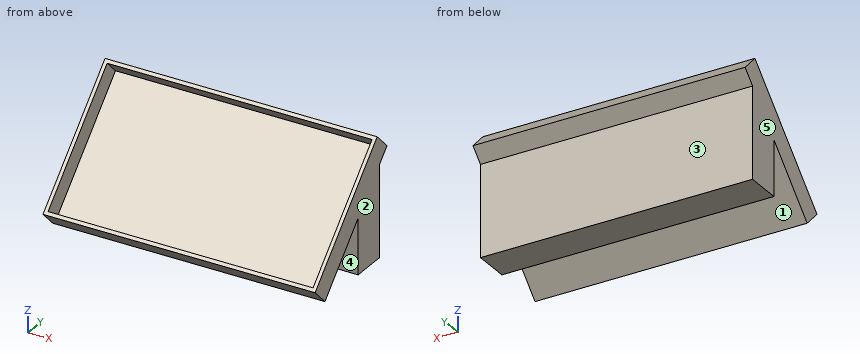
from build123d import *

# Parameters (mm, degrees)
F1_DEPTH = 152
F2_T     = -2
F4_DEPTH = 152


with BuildPart() as f1:
    # F0 (on Right) → F1 (new body)
    with BuildSketch(Plane.YZ):
        Polygon((24.395184, 33.587572), (-33.587572, -24.395184), (-24.395184, -33.587572), (33.587572, 24.395184), align=None)
    extrude(amount=F1_DEPTH)

    # F2
    f2_openings = [f1.faces().sort_by_distance(p)[0] for p in [
        (76, -4.596194, 4.596194),
    ]]
    offset(amount=F2_T, openings=f2_openings)

    # F3 (on Right) → F4 (join)
    with BuildSketch(Plane.YZ):
        Polygon((7.990418, 0), (6.604816, 0), (6.604816, -33.587572), (26.604816, -33.587572), (26.604816, 0), align=None)
        Polygon((26.604816, 18.73309), (7.990418, 0), (26.604816, 0), align=None)
    extrude(amount=F4_DEPTH)


solid = f1.part
Could you check a few things on this model? Use its own coordinates, in mm. Face numbers are marked on the shaded views. A direction names the side the tool comes from. Give positions to 0.01 mm unless a question says otherwise; leave off trailing zeros. Order: outer loops, then holes, each group sorted by start corner. A loop starts at its lowest first (then second) coordinate and runs counter-clockwise, first axis right, second up. Notation, with made-up numbers: (-21, 78.5) - (-4, 78.5) arc R23 cw to (-4, 90.5) - close; hole circle Ø5 at (14, 27.25). An arc over 180 degrees is marked (long way). One line per item, written item: value. Start each with the question number.
1. Thinking about a two-plate mould opening in Y: for the marked faces 1, 2 and 3, which applies, +Y half, -Y half, draft (parallel to the pull), parting line (faces both ways), or undercut?
2. For P1, Ø1.5, axis at x = 133, y = -18.5, coming from the +Z side; P2, Ø10, axis at x = 72.5, y = 6.5, coming from the +Z side; P3, Ø4, axis at x = 37.5, z = -9, coming from the +Y side, each with a flat end and sliding along its axis, tell me the tip position at first contact or that it passes through.
3. Imagine slicing it at B-B on x = 112.5. List the corners of the cut face in (y, z) for me, plus the area to 3 significant figures.
4. If I drill on probe 1 along X at (y, z) = (12.5, 19); probe 2 along Y at (x, z) = (99, -26); probe 3 along Z at (x, y) = (127.5, 27), over which ranges is the centre line in solid material (lowest first)?
5. Imagine slicing it at D-D on y = 16.5. List the corners of the cut face in (x, z) for me.
6. Imagine slicing it at C-C on z = 21. List the corners of the cut face in (x, y) for me, plus the area to 3 significant figures.
7. For the marked faces 4 and 5, which set-ups out of +Z, -Z, +X, -X, +Y, -Y let a thin tool reach every point of the face, with its end or its side?
8. Imagine slicing it at A-A on z = -11.5. List the corners of the cut face in (x, y) for me, plus the area to 3 significant figures.
Values:
1. face 1: undercut
1. face 2: draft
1. face 3: +Y half
2. P1: z = -24.11
2. P2: z = 5.14
2. P3: y = 26.6
3. outline: (-33.59, -24.4) - (-24.4, -33.59) - (6.6, -2.59) - (6.6, -33.59) - (26.6, -33.59) - (26.6, 17.41) - (33.59, 24.4) - (24.4, 33.59) - (22.98, 32.17) - (30.76, 24.4) - (-24.4, -30.76) - (-32.17, -22.98) - close
3. area: 1,030 mm²
4. probe 1: 0 to 2, 150 to 152
4. probe 2: -31.98 to -29.15, -19.64 to -16.81, 6.6 to 26.6
4. probe 3: 17.81 to 20.64, 28.15 to 30.98
5. outline: (0, -33.59) - (152, -33.59) - (152, 25.69) - (150, 25.69) - (150, 10.14) - (2, 10.14) - (2, 25.69) - (0, 25.69) - close
6. outline: (0, 11.81) - (2, 11.81) - (2, 27.36) - (150, 27.36) - (150, 11.81) - (152, 11.81) - (152, 30.19) - (0, 30.19) - close
6. area: 492 mm²
7. face 4: -Z, +X, -X
7. face 5: +Z, -Z, -X, +Y, -Y
8. outline: (0, -20.69) - (2, -20.69) - (2, -5.14) - (150, -5.14) - (150, -20.69) - (152, -20.69) - (152, -2.31) - (0, -2.31) - close; (0, 6.6) - (152, 6.6) - (152, 26.6) - (0, 26.6) - close
8. area: 3,530 mm²
